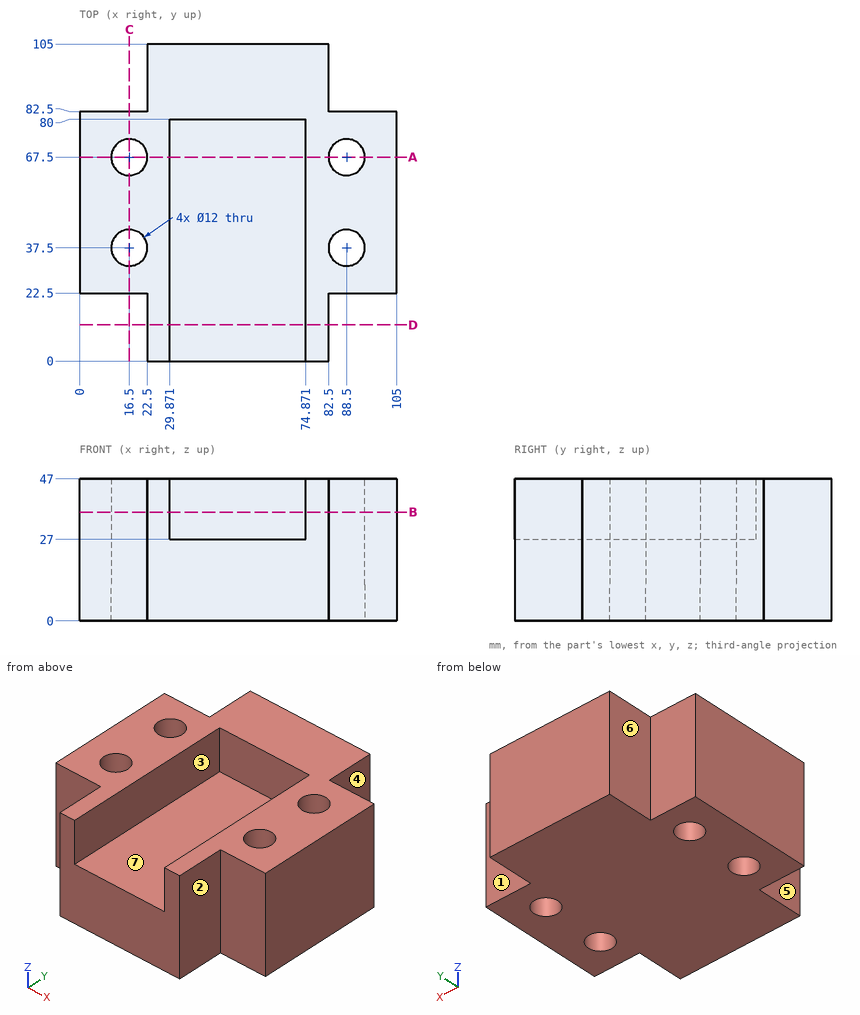
Can you work these out from the drawing? Everything is in mm from the part's minimum corner. A direction names the side the tool comes from. Give positions to 0.01 mm unless a question says otherwise; leave off trailing zeros. Loops run counter-clockwise (first coordinate to the right, second up) from the corner with the lowest first, then second, coordinate; pieces in that order, holes last. Notation, with made-up numbers: (-11, 21.5) -> (21, 21.5) arc R29 ccw to (21, 54.5) -> close; hole circle Ø10 at (-8.75, 38.5). An arc over 180 degrees is marked (long way). Write item = value, one per line.
1) Suppose I cut it at A-A on y = 67.5. Write out the boundary of the cut face in (x, z).
Check result:
outline = (0, 0) -> (10.5, 0) -> (10.5, 47) -> (0, 47) -> close; (22.5, 0) -> (82.5, 0) -> (82.5, 47) -> (74.87, 47) -> (74.87, 27) -> (29.87, 27) -> (29.87, 47) -> (22.5, 47) -> close; (94.5, 0) -> (105, 0) -> (105, 47) -> (94.5, 47) -> close
2) I need wall thicknesses on L1, parallel to Y at x = 16.5, z = 24; L2, parallel to X at y = 67, z = 25; L3, parallel to X at y = 7.5, z = 44.5. Which ranges of each line are inside material? Lowest first, please. Write a range as from..to.
Check result:
L1 = 22.5..31.5, 43.5..61.5, 73.5..82.5
L2 = 0..10.52, 22.48..82.52, 94.48..105
L3 = 22.5..29.87, 74.87..82.5
3) For the marked faces 4, 5, 6 and 7, which set-ups out of +Z, -Z, +X, -X, +Y, -Y let a thin tool reach every point of the face, with its end or its side?
Check result:
face_4 = +Z, -Z, +X, +Y
face_5 = +Z, -Z, -X, -Y
face_6 = +Z, -Z, -X, +Y
face_7 = +Z, -Y
4) Suppose I cut it at D-D on y = 12. Write out the boundary of the cut face in (x, z).
Check result:
outline = (22.5, 0) -> (82.5, 0) -> (82.5, 47) -> (74.87, 47) -> (74.87, 27) -> (29.87, 27) -> (29.87, 47) -> (22.5, 47) -> close
5) Will these pins go through, and if not, where does the flat tip stop? pin 1 (25 mm diameter, centred on x = 94.5, z = 23, fed in from -Y); pin 2 (12 mm diameter, centred on x = 89, z = 33, fed in from -Y); pin 3 (6 mm diameter, centred on x = 52.5, z = 40.5, fed in from -Y); pin 4 (7 mm diameter, centred on y = 13, z = 21, fed in from +X).
Check result:
pin_1 = 0
pin_2 = 22.5
pin_3 = 80
pin_4 = 82.5
6) Suppose I cut it at C-C on x = 16.5. Write out the boundary of the cut face in (y, z), then the cut area to 3 significant figures.
Check result:
outline = (22.5, 0) -> (31.5, 0) -> (31.5, 47) -> (22.5, 47) -> close; (43.5, 0) -> (61.5, 0) -> (61.5, 47) -> (43.5, 47) -> close; (73.5, 0) -> (82.5, 0) -> (82.5, 47) -> (73.5, 47) -> close
area = 1,690 mm2
7) Suppose I cut it at B-B on z = 36. Write out the boundary of the cut face in (x, y), then the cut area to 3 significant figures.
Check result:
outline = (0, 22.5) -> (22.5, 22.5) -> (22.5, 0) -> (29.87, 0) -> (29.87, 80) -> (74.87, 80) -> (74.87, 0) -> (82.5, 0) -> (82.5, 22.5) -> (105, 22.5) -> (105, 82.5) -> (82.5, 82.5) -> (82.5, 105) -> (22.5, 105) -> (22.5, 82.5) -> (0, 82.5) -> close; hole circle Ø12 at (16.5, 37.5); hole circle Ø12 at (16.5, 67.5); hole circle Ø12 at (88.5, 37.5); hole circle Ø12 at (88.5, 67.5)
area = 4,950 mm2
8) Thinking about a two-plate mould opening in X: for the marked faces 1, 2 and 3, which applies, released by +X, released by -X, zero draft, split by the parting line, or undercut?
Check result:
face_1 = zero draft
face_2 = released by +X
face_3 = undercut
